```python
from build123d import *

# Parameters (mm, degrees)
SKETCH1_W           = 37.5
SKETCH1_H           = 61
BOSS_EXTRUDE1_DEPTH = 1.75
SKETCH2_W           = 34.1
SKETCH2_H           = 57
BOSS_EXTRUDE2_DEPTH = 1.75
SKETCH3_W           = 31.6
SKETCH3_H           = 54.5
CUT_EXTRUDE1_DEPTH  = 1.75
CUT_EXTRUDE3_DEPTH  = 1.75
FILLET1_R           = 2.5
FILLET2_R           = 2.5
FILLET3_R           = 2.5
FILLET4_R           = 2.5


with BuildPart() as part:
    # Sketch1 → Boss-Extrude1 (new body)
    with BuildSketch(Plane(origin=(0, 0, 0), x_dir=(1, 0, 0), z_dir=(0, 1, 0))):
        with Locations((-156.892564619, -93.568616843)):
            Rectangle(SKETCH1_W, SKETCH1_H)
    extrude(amount=BOSS_EXTRUDE1_DEPTH)

    # Sketch2 → Boss-Extrude2 (add)
    with BuildSketch(Plane(origin=(0, 1.75, 0), x_dir=(1, 0, 0), z_dir=(0, 1, 0))):
        with Locations((-156.892564619, -93.568616843)):
            Rectangle(SKETCH2_W, SKETCH2_H)
    extrude(amount=BOSS_EXTRUDE2_DEPTH)

    # Sketch3 → Cut-Extrude1 (cut)
    with BuildSketch(Plane(origin=(0, 3.5, 0), x_dir=(1, 0, 0), z_dir=(0, 1, 0))):
        with Locations((-156.892564619, -93.568616843)):
            Rectangle(SKETCH3_W, SKETCH3_H)
    extrude(amount=-CUT_EXTRUDE1_DEPTH, mode=Mode.SUBTRACT)

    # Sketch4 → Cut-Extrude3 (cut)
    with BuildSketch(Plane(origin=(0, 1.75, 0), x_dir=(1, 0, 0), z_dir=(0, 1, 0))):
        with BuildLine():
            Line((-168.906040513, -118.818616843), (-144.860961832, -118.818616843))
            ThreePointArc((-144.860961832, -118.818616843), (-143.446748269, -118.232830406), (-142.860961832, -116.818616843))
            Line((-142.860961832, -116.818616843), (-142.860961832, -115.818616843))
            ThreePointArc((-142.860961832, -115.818616843), (-143.446748269, -114.404403281), (-144.860961832, -113.818616843))
            Line((-144.860961832, -113.818616843), (-168.906040513, -113.818616843))
            ThreePointArc((-168.906040513, -113.818616843), (-170.320254075, -114.404403281), (-170.906040513, -115.818616843))
            Line((-170.906040513, -115.818616843), (-170.906040513, -116.818616843))
            ThreePointArc((-170.906040513, -116.818616843), (-170.320254075, -118.232830406), (-168.906040513, -118.818616843))
        make_face()
        with BuildLine():
            Line((-168.906040513, -103.818616843), (-144.860961832, -103.818616843))
            ThreePointArc((-144.860961832, -103.818616843), (-143.446748269, -103.232830406), (-142.860961832, -101.818616843))
            Line((-142.860961832, -101.818616843), (-142.860961832, -100.818616843))
            ThreePointArc((-142.860961832, -100.818616843), (-143.446748269, -99.404403281), (-144.860961832, -98.818616843))
            Line((-144.860961832, -98.818616843), (-168.906040513, -98.818616843))
            ThreePointArc((-168.906040513, -98.818616843), (-170.320254075, -99.404403281), (-170.906040513, -100.818616843))
            Line((-170.906040513, -100.818616843), (-170.906040513, -101.818616843))
            ThreePointArc((-170.906040513, -101.818616843), (-170.320254075, -103.232830406), (-168.906040513, -103.818616843))
        make_face()
        with BuildLine():
            Line((-168.906040513, -96.318616843), (-144.860961832, -96.318616843))
            ThreePointArc((-144.860961832, -96.318616843), (-143.446748269, -95.732830406), (-142.860961832, -94.318616843))
            Line((-142.860961832, -94.318616843), (-142.860961832, -93.318616843))
            ThreePointArc((-142.860961832, -93.318616843), (-143.446748269, -91.904403281), (-144.860961832, -91.318616843))
            Line((-144.860961832, -91.318616843), (-168.906040513, -91.318616843))
            ThreePointArc((-168.906040513, -91.318616843), (-170.320254075, -91.904403281), (-170.906040513, -93.318616843))
            Line((-170.906040513, -93.318616843), (-170.906040513, -94.318616843))
            ThreePointArc((-170.906040513, -94.318616843), (-170.320254075, -95.732830406), (-168.906040513, -96.318616843))
        make_face()
        with BuildLine():
            Line((-168.906040513, -81.318616843), (-144.860961832, -81.318616843))
            ThreePointArc((-144.860961832, -81.318616843), (-143.446748269, -80.732830406), (-142.860961832, -79.318616843))
            Line((-142.860961832, -79.318616843), (-142.860961832, -78.318616843))
            ThreePointArc((-142.860961832, -78.318616843), (-143.446748269, -76.904403281), (-144.860961832, -76.318616843))
            Line((-144.860961832, -76.318616843), (-168.906040513, -76.318616843))
            ThreePointArc((-168.906040513, -76.318616843), (-170.320254075, -76.904403281), (-170.906040513, -78.318616843))
            Line((-170.906040513, -78.318616843), (-170.906040513, -79.318616843))
            ThreePointArc((-170.906040513, -79.318616843), (-170.320254075, -80.732830406), (-168.906040513, -81.318616843))
        make_face()
        with BuildLine():
            Line((-168.906040513, -111.318616843), (-144.860961832, -111.318616843))
            ThreePointArc((-144.860961832, -111.318616843), (-143.446748269, -110.732830406), (-142.860961832, -109.318616843))
            Line((-142.860961832, -109.318616843), (-142.860961832, -108.318616843))
            ThreePointArc((-142.860961832, -108.318616843), (-143.446748269, -106.904403281), (-144.860961832, -106.318616843))
            Line((-144.860961832, -106.318616843), (-168.906040513, -106.318616843))
            ThreePointArc((-168.906040513, -106.318616843), (-170.320254075, -106.904403281), (-170.906040513, -108.318616843))
            Line((-170.906040513, -108.318616843), (-170.906040513, -109.318616843))
            ThreePointArc((-170.906040513, -109.318616843), (-170.320254075, -110.732830406), (-168.906040513, -111.318616843))
        make_face()
        with BuildLine():
            Line((-168.906040513, -88.818616843), (-144.860961832, -88.818616843))
            ThreePointArc((-144.860961832, -88.818616843), (-143.446748269, -88.232830406), (-142.860961832, -86.818616843))
            Line((-142.860961832, -86.818616843), (-142.860961832, -85.818616843))
            ThreePointArc((-142.860961832, -85.818616843), (-143.446748269, -84.404403281), (-144.860961832, -83.818616843))
            Line((-144.860961832, -83.818616843), (-168.906040513, -83.818616843))
            ThreePointArc((-168.906040513, -83.818616843), (-170.320254075, -84.404403281), (-170.906040513, -85.818616843))
            Line((-170.906040513, -85.818616843), (-170.906040513, -86.818616843))
            ThreePointArc((-170.906040513, -86.818616843), (-170.320254075, -88.232830406), (-168.906040513, -88.818616843))
        make_face()
        with BuildLine():
            Line((-168.906040513, -73.818616843), (-144.860961832, -73.818616843))
            ThreePointArc((-144.860961832, -73.818616843), (-143.446748269, -73.232830406), (-142.860961832, -71.818616843))
            Line((-142.860961832, -71.818616843), (-142.860961832, -70.818616843))
            ThreePointArc((-142.860961832, -70.818616843), (-143.446748269, -69.404403281), (-144.860961832, -68.818616843))
            Line((-144.860961832, -68.818616843), (-168.906040513, -68.818616843))
            ThreePointArc((-168.906040513, -68.818616843), (-170.320254075, -69.404403281), (-170.906040513, -70.818616843))
            Line((-170.906040513, -70.818616843), (-170.906040513, -71.818616843))
            ThreePointArc((-170.906040513, -71.818616843), (-170.320254075, -73.232830406), (-168.906040513, -73.818616843))
        make_face()
    extrude(amount=-CUT_EXTRUDE3_DEPTH, mode=Mode.SUBTRACT)

    # Fillet1
    fillet1_edges = [part.edges().sort_by_distance(p)[0] for p in [
        (-138.142564619, 0.875, 63.068616843),
    ]]
    fillet(fillet1_edges, radius=FILLET1_R)

    # Fillet2
    fillet2_edges = [part.edges().sort_by_distance(p)[0] for p in [
        (-175.642564619, 0.875, 63.068616843),
    ]]
    fillet(fillet2_edges, radius=FILLET2_R)

    # Fillet3
    fillet3_edges = [part.edges().sort_by_distance(p)[0] for p in [
        (-175.642564619, 0.875, 124.068616843),
    ]]
    fillet(fillet3_edges, radius=FILLET3_R)

    # Fillet4
    fillet4_edges = [part.edges().sort_by_distance(p)[0] for p in [
        (-138.142564619, 0.875, 124.068616843),
    ]]
    fillet(fillet4_edges, radius=FILLET4_R)


solid = part.part
```
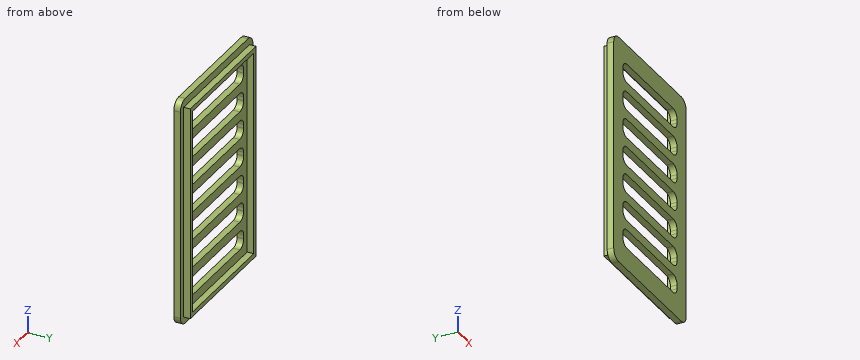
Here's how the part is built. I have some questions about the finished solid (model axes, mm). Give positions to 0.01 mm unless a question says otherwise; leave off trailing zeros. Loops run counter-clockwise (first coordinate to the right, second up) from the corner with the lowest first, then second, coordinate; pieces in that order, holes last. Notation, with made-up numbers: M 21.25,-1 L 31.25,-1 A23 ccw 31.25,11 Z; hole C 14,63 d10. An arc over 180 degrees is marked long. Put each result on its own line as item: value. Start each with the question number.
(1) I want a section at A-A on z = 75.5. Please give me the cut outline in (x, y).
(2) Will these pins go through, and if not, where does the flat tip stop? pin 1 Ø1.4 at (y, z) = (3, 106.5) entering from +X; pin 2 Ø10 at (x, z) = (-148.5, 95.5) entering from +Y; pin 3 Ø2 at (x, y) = (-147, 3) entering from -Z.
(3) I want a section at B-B on y = 2.85. Please give me the cut outline in (x, z).
(4) I want a section at D-D on x = -162.5. State how many separate pieces and enclosed holes the cut face has, then the cut area to 3 significant figures.
(5) I need wall thicknesses on line 1 along X through (y, z) = (3.35, 101); line 2 along Z through (x, y) = (-168, 2.95); line 3 along X through (y, z) = (0.5, 71.5). Which ranges of each line are inside material? Lowest first, please. Write a range as [from, to].
(6) I want a section at C-C on z = 95.5. Please give me the cut outline in (x, y), then the cut area to 3 significant figures.
Answer block:
1. outline: M -175.64,0 L -138.14,0 L -138.14,1.75 L -139.84,1.75 L -139.84,3.5 L -141.09,3.5 L -141.09,1.75 L -172.69,1.75 L -172.69,3.5 L -173.94,3.5 L -173.94,1.75 L -175.64,1.75 Z
2. pin 1: x = -139.84
2. pin 2: y = 1.75
2. pin 3: z = 65.07
3. outline: M -173.94,65.07 L -139.84,65.07 L -139.84,122.07 L -173.94,122.07 Z; hole M -172.69,66.32 L -141.09,66.32 L -141.09,120.82 L -172.69,120.82 Z
4. separate pieces: 8
4. enclosed holes: 0
4. area: 49.9 mm^2
5. line 1: [-173.94, -172.69], [-141.09, -139.84]
5. line 2: [65.07, 66.32], [120.82, 122.07]
5. line 3: [-175.64, -170.91], [-142.86, -138.14]
6. outline: M -175.64,0 L -170.52,0 L -170.52,1.75 L -172.69,1.75 L -172.69,3.5 L -173.94,3.5 L -173.94,1.75 L -175.64,1.75 Z; M -143.25,0 L -138.14,0 L -138.14,1.75 L -139.84,1.75 L -139.84,3.5 L -141.09,3.5 L -141.09,1.75 L -143.25,1.75 Z
6. area: 22.3 mm^2
